CAD build for the part. Positions are in the model's coordinates, mm. Face numbers are marked on the shaded views. A direction names the side the tool comes from. Round coordinates to 2 decimals unless told otherwise and drop trailing zeros. Order: outer loops, then holes, each group sorted by start corner. A loop starts at its lowest first (then second) coordinate and runs counter-clockwise, first axis right, second up. Notation, with made-up numbers: M 0,-19 L 17,-19 A10 ccw 17,-9 Z; hole C -10.75,78.5 d11. An arc over 180 degrees is marked long. Answer as a JSON object with one key per item and string values.
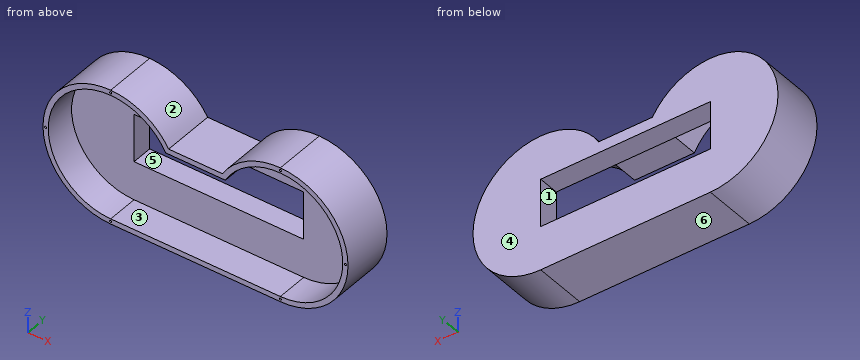
Autodesk Inventor part; units mm, degrees
ref_plane "Work Plane1" through (0, -25, 0) normal (0, -1, 0) x (1, 0, 0)
ref_plane "YZ Plane" through (0, 0, 0) normal (1, 0, 0) x (0, 1, 0)
ref_plane "XZ Plane" through (0, 0, 0) normal (0, 1, 0) x (-1, 0, 0)
sketch "Sketch1" plane through (0, 0, 0) normal (0, 1, 0) x (-1, 0, 0)
  line L0 (0, 0) -> (0, -22.1379) construction
  line L1 (0, 0) -> (0, 22.1379) construction
  line L2 (0, 0) -> (40.725, 0) construction
  line L3 (0, 0) -> (-40.725, 0) construction
  circle A0 centre (-40.725, 0) radius 30 construction
  circle A1 centre (-40.725, 0) radius 32.5 construction
  circle A2 centre (40.725, 0) radius 30 construction
  circle A3 centre (40.725, 0) radius 32.5 construction
  line L4 (40.725, -30) -> (40.725, 30) construction
  line L5 (40.725, -30) -> (40.725, -32.5) construction
  line L6 (40.725, 30) -> (40.725, 32.5) construction
  line L7 (-40.725, 30) -> (-40.725, -30) construction
  line L8 (-40.725, -32.5) -> (-40.725, -30) construction
  line L9 (-40.725, 30) -> (-40.725, 32.5) construction
  line L10 (40.725, -32.5) -> (-40.725, -32.5) construction
  line L11 (40.725, -30) -> (-40.725, -30) construction
  line L12 (40.725, 32.5) -> (40.725, 14.2758) construction
  line L13 (40.725, 14.2758) -> (-40.725, 14.2758) construction
  line L14 (40.725, 32.5) -> (40.725, 16.7758) construction
  line L15 (40.725, 16.7758) -> (-40.725, 16.7758) construction
  arc A4 (40.725, -30) -> (70.725, 0) centre (40.725, 0) ccw
  arc A5 (70.725, 0) -> (40.725, 30) centre (40.725, 0) ccw
  arc A6 (40.725, 32.5) -> (12.8894, 16.7758) centre (40.725, 0) ccw
  arc A7 (73.225, 0) -> (40.725, 32.5) centre (40.725, 0) ccw
  arc A8 (40.725, -32.5) -> (73.225, 0) centre (40.725, 0) ccw
  line L16 (40.725, -30) -> (-40.725, -30)
  line L17 (-40.725, -32.5) -> (40.725, -32.5)
  line L18 (12.8894, 16.7758) -> (-12.8894, 16.7758)
  line L19 (14.3394, 14.2758) -> (-14.3394, 14.2758)
  arc A9 (40.725, 30) -> (14.3394, 14.2758) centre (40.725, 0) ccw
  arc A10 (-12.8894, 16.7758) -> (-40.725, 32.5) centre (-40.725, 0) ccw
  arc A11 (-14.3394, 14.2758) -> (-40.725, 30) centre (-40.725, 0) ccw
  arc A12 (-40.725, 30) -> (-70.725, 0) centre (-40.725, 0) ccw
  arc A13 (-40.725, 32.5) -> (-73.225, 0) centre (-40.725, 0) ccw
  arc A14 (-70.725, 0) -> (-40.725, -30) centre (-40.725, 0) ccw
  arc A15 (-73.225, 0) -> (-40.725, -32.5) centre (-40.725, 0) ccw
  line L20 (0, 0) -> (39, 0) construction
  line L21 (0, 0) -> (-39, 0) construction
  line L22 (40.725, 0) -> (40.725, -11.5) construction
  line L23 (40.725, 0) -> (40.725, 11.5) construction
  line L24 (-40.725, 0) -> (-40.725, -11.5) construction
  line L25 (-40.725, 0) -> (-40.725, 11.5) construction
  line L26 (40.725, -11.5) -> (-40.725, -11.5)
  line L27 (40.725, 11.5) -> (-40.725, 11.5)
  line L28 (-40.725, 11.5) -> (-40.725, -11.5)
  line L29 (40.725, -11.5) -> (40.725, 11.5)
  dimension "d0" = 22.1379
  dimension "d1" = 22.1379
  dimension "d2" = 40.725
  dimension "d3" = 40.725
  dimension "d4" = 60
  dimension "d5" = 65
  dimension "d6" = 60
  dimension "d7" = 65
  dimension "d8" = 18.2242
  dimension "d9" = 15.7241
  dimension "d10" = 39
  dimension "d11" = 39
  dimension "d12" = 11.5
  dimension "d13" = 11.5
  dimension "d14" = 11.5
  dimension "d15" = 11.5
extrude "Extrusion1" add sketch "Sketch1" against normal blind 10 contours L16 A14 A12 A11 L19 A9 A5 A4
extrude "Extrusion2" add sketch "Sketch1" against normal blind 25 contours A7 A8 L17 A15 A13 A10 L18 A6
ref_plane "Work Plane1" through (0, -25, 0) normal (0, -1, 0) x (1, 0, 0)
sketch "Sketch2" plane through (0, -25, 0) normal (0, -1, 0) x (1, 0, 0)
  arc A0 (-14.3394, 14.2758) -> (-40.725, -30) centre (-40.725, 0) ccw
  arc A1 (-12.8894, 16.7758) -> (-40.725, -32.5) centre (-40.725, 0) ccw
  arc A2 (40.725, -32.5) -> (12.8894, 16.7758) centre (40.725, 0) ccw
  arc A3 (40.725, -30) -> (14.3394, 14.2758) centre (40.725, 0) ccw
  line L0 (-14.3394, 14.2758) -> (14.3394, 14.2758)
  line L1 (12.8894, 16.7758) -> (-12.8894, 16.7758)
  line L2 (40.725, -30) -> (-40.725, -30)
  line L3 (-40.725, -32.5) -> (40.725, -32.5)
  line L4 (-40.725, 30) -> (-40.725, -30) construction
  line L5 (-40.725, 30) -> (-40.725, 32.5) construction
  line L6 (-40.725, -30) -> (-40.725, -32.5) construction
  line L7 (40.725, 30) -> (40.725, -30) construction
  line L8 (40.725, 30) -> (40.725, 32.5) construction
  line L9 (40.725, -30) -> (40.725, -32.5) construction
  line L10 (-70.725, 0) -> (70.725, 0) construction
  line L11 (70.725, 0) -> (73.225, 0) construction
  line L12 (-73.225, 0) -> (-70.725, 0) construction
  line L13 (0, 14.2758) -> (0, -30) construction
  line L14 (0, -30) -> (0, -32.5) construction
  line L15 (0, 14.2758) -> (0, 16.7758) construction
  circle A4 centre (71.975, 0) radius 0.5
  circle A5 centre (40.725, -31.25) radius 0.5
  circle A6 centre (40.725, 31.25) radius 0.5
  circle A7 centre (0, 15.5258) radius 0.5
  circle A8 centre (-40.725, 31.25) radius 0.5
  circle A9 centre (-71.975, 0) radius 0.5
  circle A10 centre (-40.725, -31.25) radius 0.5
  point P0 (0, 0)
  dimension "d21" = 1
  dimension "d22" = 1
  dimension "d23" = 1
  dimension "d24" = 1
  dimension "d25" = 1
  dimension "d26" = 1
  dimension "d27" = 1
extrude "Extrusion3" cut sketch "Sketch2" against normal blind 1 contours A4 | A5 | A6 | A8 | A9 | A10
equation "\"d28\" = d22"
properties part number "con_v8_d1_back_3DPrint"
Item 1: Two-plate mould, pull along Z, no slides. Class the marked faces 4, 5 and 6: released by +Z, released by -Z, zero draft, split by the parting line, or undercut.
Worked answers:
{"face 4": "zero draft", "face 5": "undercut", "face 6": "released by -Z"}
Item 2: 3-axis set-ups, long thin cutter, end or side, ignore diameter. For the marked faces 1, 2 and 3: which of +Z, -Z, +X, -X, +Y, -Y reach the whole face in a straight line?
Worked answers:
{"face 1": "+Y, -Y", "face 2": "+Z, +Y, -Y", "face 3": "-Y"}
Item 3: Saw through at B-B on y = -3. List the corners of the cut face in (x, z) (3 decimals), and give its area (3 significant figures).
Worked answers:
{"outline": "M -40.725,-32.5 L 40.725,-32.5 A32.5 ccw 40.725,32.5 A32.5 ccw 12.889,16.776 L -12.889,16.776 A32.5 ccw -40.725,32.5 A32.5 ccw Z; hole M -40.725,-11.5 L 40.725,-11.5 L 40.725,11.5 L -40.725,11.5 Z", "area": "6,080 mm2"}
Item 4: Saw through at C-C on z = -10. List the corners of the cut face in (x, y) (3 decimals), and give its area (3 significant figures).
Worked answers:
{"outline": "M -71.648,-25 L -69.009,-25 L -69.009,-10 L -40.725,-10 L -40.725,0 L -71.648,0 Z; M 40.725,-10 L 69.009,-10 L 69.009,-25 L 71.648,-25 L 71.648,0 L 40.725,0 Z", "area": "698 mm2"}
Item 5: Saw through at D-D on x = -55. List the corners of the cut face in (y, z), and give its area (3 significant figures).
Worked answers:
{"outline": "M -25,-29.2 L 0,-29.2 L 0,29.2 L -25,29.2 L -25,26.39 L -10,26.39 L -10,-26.39 L -25,-26.39 Z", "area": "668 mm2"}
Item 6: Saw through at A-A on x = 8. List the corners of the cut face in (y, z), and give its area (3 significant figures).
Worked answers:
{"outline": "M -25,-32.5 L 0,-32.5 L 0,-11.5 L -10,-11.5 L -10,-30 L -25,-30 Z; M -25,14.28 L -10,14.28 L -10,11.5 L 0,11.5 L 0,16.78 L -25,16.78 Z", "area": "338 mm2"}
Item 7: Drop flat-ended pins along their axis: pin 1 Ø1.5 at (x, z) = (-33.5, 21.5) entering from -Y; pin 2 Ø1.5 at (y, z) = (-20, 24) entering from -X; pin 3 Ø12 at (x, y) = (58.5, -11.5) entering from -Z. Give the stop position or say it passes through.
Worked answers:
{"pin 1": "stops at y = -10", "pin 2": "stops at x = -63.43", "pin 3": "stops at z = -30.29"}
Item 8: Wall check: line 1 along Z through (x, y) = (-10, -22.75); line 2 along Z through (x, y) = (-41, -12); line 3 along X through (y, z) = (-18, 27) (3 decimals). Give the ranges that are in metal, low to high. Write a range as [from, to].
Worked answers:
{"line 1": "z = [-32.5, -30], [14.28, 16.78]", "line 2": "z = [-32.5, -30], [30, 32.5]", "line 3": "x = [-58.815, -53.802], [-27.648, -22.635], [22.635, 27.648], [53.802, 58.815]"}
